Work out the finished part from the listing and answer in its coordinate system (mm). A direction names the side the tool comes from. Give positions to 0.01 mm unless a question says otherwise; leave off trailing zeros. Order: outer loops, then holes, each group sorted by start corner. A loop starts at its lowest first (then second) coordinate and runs counter-clockwise, first axis right, second up. Notation, with made-up numbers: (70, -1.5) - (86, -1.5) arc R11 cw to (86, 15.5) - close; hole circle Ø5 at (-26, 38). An arc over 180 degrees is marked (long way). Put each result on its own line as item: value.
```python
from build123d import *

# Parameters (mm, degrees)
SKETCH_1_W          = 127.8
SKETCH_1_H          = 7.8
EXTRUDE_1_DEPTH     = 9.6
SKETCH_2_R          = 2.4
EXTRUDE_2_DEPTH     = 1.7
SKETCH_3_R          = 2.962272449
CUT_EXTRUDE_1_DEPTH = 1.8


with BuildPart() as part:
    # Эскиз1 → Бобышка-Вытянуть1 (new body)
    with BuildSketch(Plane.XY):
        Rectangle(SKETCH_1_W, SKETCH_1_H)
    extrude(amount=EXTRUDE_1_DEPTH)

    # Эскиз2 → Бобышка-Вытянуть2 (add)
    with BuildSketch(Plane(origin=(0, 0, 0), x_dir=(-1, 0, 0), z_dir=(0, 0, -1))):
        with Locations((-60, 0)):
            Circle(SKETCH_2_R)
        with Locations((-52, 0)):
            Circle(SKETCH_2_R)
        with Locations((-44, 0)):
            Circle(SKETCH_2_R)
        with Locations((-36, 0)):
            Circle(SKETCH_2_R)
        with Locations((-28, 0)):
            Circle(SKETCH_2_R)
        with Locations((-20, 0)):
            Circle(SKETCH_2_R)
        with Locations((-12, 0)):
            Circle(SKETCH_2_R)
        with Locations((-4, 0)):
            Circle(SKETCH_2_R)
        with Locations((4, 0)):
            Circle(SKETCH_2_R)
        with Locations((12, 0)):
            Circle(SKETCH_2_R)
        with Locations((20, 0)):
            Circle(SKETCH_2_R)
        with Locations((28, 0)):
            Circle(SKETCH_2_R)
        with Locations((36, 0)):
            Circle(SKETCH_2_R)
        with Locations((44, 0)):
            Circle(SKETCH_2_R)
        with Locations((52, 0)):
            Circle(SKETCH_2_R)
        with Locations((60, 0)):
            Circle(SKETCH_2_R)
    extrude(amount=EXTRUDE_2_DEPTH)

    # Эскиз3 → Вырез-Вытянуть1 (cut)
    with BuildSketch(Plane.XY.offset(9.6)):
        with Locations((60, 0)):
            Circle(SKETCH_3_R)
        with Locations((52, 0)):
            Circle(SKETCH_3_R)
        with Locations((44, 0)):
            Circle(SKETCH_3_R)
        with Locations((36, 0)):
            Circle(SKETCH_3_R)
        with Locations((28, 0)):
            Circle(SKETCH_3_R)
        with Locations((20, 0)):
            Circle(SKETCH_3_R)
        with Locations((12, 0)):
            Circle(SKETCH_3_R)
        with Locations((4, 0)):
            Circle(SKETCH_3_R)
        with Locations((-4, 0)):
            Circle(SKETCH_3_R)
        with Locations((-12, 0)):
            Circle(SKETCH_3_R)
        with Locations((-20, 0)):
            Circle(SKETCH_3_R)
        with Locations((-28, 0)):
            Circle(SKETCH_3_R)
        with Locations((-36, 0)):
            Circle(SKETCH_3_R)
        with Locations((-44, 0)):
            Circle(SKETCH_3_R)
        with Locations((-52, 0)):
            Circle(SKETCH_3_R)
        with Locations((-60, 0)):
            Circle(SKETCH_3_R)
    extrude(amount=-CUT_EXTRUDE_1_DEPTH, mode=Mode.SUBTRACT)


solid = part.part
```
(1) A tool of negligible diameter and unlimited length cuts with its end or side. For faces 5 (the face through (-36, 0, -1.7)), 6 (the face through (38.74, -1.13, 8.71)), 7 (the face through (-41.602, 0.106, -0.838)), from which of +Z, -Z, +X, -X, +Y, -Y can it reach the whole face along a straight path? Write none if from no direction.
Geometry check:
face 5: -Z, +X, -X, +Y, -Y
face 6: +Z
face 7: -Z
(2) Section B-B, the plane x = -37 is taken. Write down the section's boundary in (y, z).
Geometry check:
outline: (-3.9, 0) - (-2.18, 0) - (-2.18, -1.7) - (2.18, -1.7) - (2.18, 0) - (3.9, 0) - (3.9, 9.6) - (2.79, 9.6) - (2.79, 7.8) - (-2.79, 7.8) - (-2.79, 9.6) - (-3.9, 9.6) - close
(3) Determine the mould class of faces 1 (the face through (12, 0, -1.7)), 2 (the face through (60, 0, 7.8)), 3 (the face through (25.71, 0.72, -0.84)), 4 (the face through (-1.26, -1.13, 8.71)) for opening direction Y: pulls with the +Y half, pulls with the -Y half, needs draft (parallel to the pull), parting line crosses it, or undercut.
Geometry check:
face 1: needs draft
face 2: undercut
face 3: parting line crosses it
face 4: undercut
(4) Given pin 1 (1.8 mm diameter, centred on x = 61, y = 0, fed in from +Z), flat-ended and moving along its own axis, determine where the tip first touches the part or whether it passes through.
Geometry check:
pin 1: stops at z = 7.8
(5) Straight lines are drawn through the part: line 1 (Y direction, x = -44, z = 8.9); line 2 (Z direction, x = -44.5, y = 1); line 3 (Z direction, x = 28.5, y = 2.5). For each, find the intervals that lie inside material, in ascending order.
Geometry check:
line 1: y = -3.9 to -2.96, 2.96 to 3.9
line 2: z = -1.7 to 7.8
line 3: z = 0 to 7.8
(6) Section A-A, the plane x = -12 is taken. Write down the section's boundary in (y, z), then the cut area to 3 significant figures.
Geometry check:
outline: (-3.9, 0) - (-2.4, 0) - (-2.4, -1.7) - (2.4, -1.7) - (2.4, 0) - (3.9, 0) - (3.9, 9.6) - (2.96, 9.6) - (2.96, 7.8) - (-2.96, 7.8) - (-2.96, 9.6) - (-3.9, 9.6) - close
area: 72.4 mm²
